```python
from build123d import *

# Parameters (mm, degrees)
SKETCH1_R             = 11.5
SKETCH1_R_2           = 10
SKETCH1_R_3           = 2
BOSS_EXTRUDE1_DEPTH   = 7
SKETCH2_R             = 11
CUT_EXTRUDE1_DEPTH    = 6
M4_TAPPED_HOLE1_D     = 3.3
M4_TAPPED_HOLE1_DEPTH = 5
M4_TAPPED_HOLE1_TIP   = 0.991420021


with BuildPart() as part:
    # Sketch1 → Boss-Extrude1 (new body)
    with BuildSketch(Plane(origin=(0, 0, 0), x_dir=(1, 0, 0), z_dir=(0, 1, 0))):
        with BuildLine():
            Line((150, -15), (-150, -15))
            ThreePointArc((-150, -15), (-165, 0), (-150, 15))
            Line((-150, 15), (150, 15))
            ThreePointArc((150, 15), (165, 0), (150, -15))
        make_face()
        with Locations(Location((150, 0, 0), (0, 0, 270))):
            Circle(SKETCH1_R, mode=Mode.SUBTRACT)
        with Locations(Location((-150, 0, 0), (0, 0, 270))):
            Circle(SKETCH1_R_2, mode=Mode.SUBTRACT)
        with Locations(Location((40.999999907, 0, 0), (0, 0, 270))):
            Circle(SKETCH1_R_3, mode=Mode.SUBTRACT)
        with Locations(Location((-40.99999998, 0, 0), (0, 0, 270))):
            Circle(SKETCH1_R_3, mode=Mode.SUBTRACT)
        with BuildLine():
            Line((109.999999927, 9), (53.999999907, 9))
            ThreePointArc((53.999999907, 9), (44.999999907, 0), (53.999999907, -9))
            Line((53.999999907, -9), (109.999999927, -9))
            ThreePointArc((109.999999927, -9), (119, 0), (109.999999927, 9))
        make_face(mode=Mode.SUBTRACT)
        with BuildLine():
            Line((27.999999907, 9), (-28.000000112, 9))
            ThreePointArc((-28.000000112, 9), (-36.99999998, 0), (-28.000000112, -9))
            Line((-28.000000112, -9), (27.999999907, -9))
            ThreePointArc((27.999999907, -9), (36.999999907, 0), (27.999999907, 9))
        make_face(mode=Mode.SUBTRACT)
        with BuildLine():
            Line((-53.99999998, 9), (-110, 9))
            ThreePointArc((-110, 9), (-119, 0), (-110, -9))
            Line((-110, -9), (-53.99999998, -9))
            ThreePointArc((-53.99999998, -9), (-44.99999998, 0), (-53.99999998, 9))
        make_face(mode=Mode.SUBTRACT)
    extrude(amount=BOSS_EXTRUDE1_DEPTH)

    # Sketch2 → Cut-Extrude1 (cut)
    with BuildSketch(Plane(origin=(0, 7, 0), x_dir=(1, 0, 0), z_dir=(0, 1, 0))):
        with Locations(Location((-150, 0, 0), (0, 0, 270))):
            Circle(SKETCH2_R)
    extrude(amount=-CUT_EXTRUDE1_DEPTH, mode=Mode.SUBTRACT)

    # M4 Tapped Hole1
    with Locations(Plane(origin=(0, 7, 0), x_dir=(1, 0, 0), z_dir=(0, 1, 0))):
        with Locations((-135, 10), (-135, -10)):
            Hole(M4_TAPPED_HOLE1_D / 2, depth=M4_TAPPED_HOLE1_DEPTH)
            with Locations((0, 0, -(M4_TAPPED_HOLE1_DEPTH + M4_TAPPED_HOLE1_TIP / 2))):  # 118° drill point
                Cone(0, M4_TAPPED_HOLE1_D / 2, M4_TAPPED_HOLE1_TIP, mode=Mode.SUBTRACT)


solid = part.part
```
Verification items for the finished model (mm, model axes). A direction names the side the tool comes from. Coordinates: 2 decimals unless noted, no trailing zeros. Write each loop counter-clockwise with the first axis right and the second up, starting at its lowest first coordinate (ties: lowest second). Pieces come first, ordered by that corner, then holes. Notation, with made-up numbers: M 33.5,61 L 40.5,61 A24 ccw 40.5,88 Z; hole C -37,39 d4. An arc over 180 degrees is marked long. Answer as a JSON object with one key per item and string values. Group by question number.
(1) Material ranges on line 1 (Z direction, x = -135, y = 6); line 2 (Z direction, x = 92.5, y = 3.25); line 3 (X direction, y = 5.5, z = -8), recorded low to high.
(2) Cross-section at B-B, the plane y = 4. State how many separate pieces and enclosed holes the cut face has, and give its area (3 significant figures).
(3) Gauge pin test, flat ends, axial feed: pin 1 (13 mm diameter, centred on x = -150, z = 0, fed in from -Y); pin 2 (12 mm diameter, centred on x = 8.5, z = -9.5, fed in from -Y); pin 3 (2.5 mm diameter, centred on x = -135, z = 10, fed in from +Y); pin 4 (2 mm diameter, centred on y = 4.5, z = -8, fed in from -X). Record the tip position at first contact, or that the pin passes through.
(4) Cross-section at C-C, the plane z = -5. Record the cut outline in (x, y).
(5) Release check for a two-part mould opening along Z. For faces 3 (the face through (-2, 3, -15)), 4 (the face through (82, 3, -9)), 5 (the face through (-165, 3, 0)) record: +Z half, -Z half, draft (parallel to the pull), parting line (faces both ways), or undercut.
(6) Cross-section at A-A, the plane x = 22. Record the cut outline in (y, z), and give its area (3 significant figures).
(7) Tool access check on faces 1 (the face through (2, 3, 15)), 2 (the face through (-119, 3, 0)). Record the directions out of +Z, -Z, +X, -X, +Y, -Y that give a thin tool (end or side, any length) a straight path to the whole face; none if there is none.
Reply:
{
 "1": {"line 1": "-15 to -11.65, -8.35 to 8.35, 11.65 to 15", "line 2": "-15 to -9, 9 to 15", "line 3": "-162.69 to -157.55, -142.45 to -114.12, -49.88 to -32.12, 32.12 to 49.88, 114.12 to 141.74, 158.26 to 162.69"},
 "2": {"separate pieces": "1", "enclosed holes": "9", "area": "5,080 mm²"},
 "3": {"pin 1": "through", "pin 2": "y = 0", "pin 3": "y = 1.76", "pin 4": "x = -163.27"},
 "4": {"outline": "M -164.14,0 L -158.66,0 L -158.66,1 L -159.8,1 L -159.8,7 L -164.14,7 Z; M -141.34,0 L -117.48,0 L -117.48,7 L -140.2,7 L -140.2,1 L -141.34,1 Z; M -46.52,0 L -35.48,0 L -35.48,7 L -46.52,7 Z; M 35.48,0 L 46.52,0 L 46.52,7 L 35.48,7 Z; M 117.48,0 L 139.64,0 L 139.64,7 L 117.48,7 Z; M 160.36,0 L 164.14,0 L 164.14,7 L 160.36,7 Z"},
 "5": {"face 3": "-Z half", "face 4": "undercut", "face 5": "parting line"},
 "6": {"outline": "M 0,-15 L 7,-15 L 7,-9 L 0,-9 Z; M 0,9 L 7,9 L 7,15 L 0,15 Z", "area": "84.0 mm²"},
 "7": {"face 1": "+Z, +X, -X, +Y, -Y", "face 2": "+Y, -Y"}
}
